Can you work these out from the model? Positions are in its coordinate system, mm. A direction names the side the tool comes from. Coordinates: 2 decimals unless noted, no trailing zeros. Order: outer loops, then holes, each group sorted by start corner. A loop starts at its lowest first (then second) coordinate and runs counter-clockwise, first axis right, second up. Notation, with made-up numbers: (-21.5, -39) -> (4.5, -39) arc R23 cw to (4.5, 0) -> close; hole circle Ø1 at (76.25, -31). An arc over 180 degrees is marked (long way). Answer as CSV lines item,"result".
from build123d import *

# Parameters (mm, degrees)
M10_TAPPED_HOLE1_D           = 8.5
M10_TAPPED_HOLE1_DEPTH       = 24.5
M10_TAPPED_HOLE1_CSINK_D     = 10.05
M10_TAPPED_HOLE1_CSINK_ANGLE = 90
M10_TAPPED_HOLE1_TIP         = 2.553657631
M10_TAPPED_HOLE2_D           = 8.5
M10_TAPPED_HOLE2_DEPTH       = 24.5
M10_TAPPED_HOLE2_CSINK_D     = 10.05
M10_TAPPED_HOLE2_CSINK_ANGLE = 90
M10_TAPPED_HOLE2_TIP         = 2.553657631
CHAMFER1_SIZE                = 1


with BuildPart() as part:
    # Sketch1 → Revolve1 (revolve)
    with BuildSketch(Plane.XY, mode=Mode.PRIVATE) as revolve1_sk:
        Polygon((0, 0), (0, 30), (53.5, 30), (53.5, 32.5), (71.5, 32.5), (71.5, 30), (188, 30), (188, 0), align=None)
    revolve(revolve1_sk.sketch.rotate(Axis((0, 0, 0), (1, 0, 0)), 90), axis=Axis((0, 0, 0), (1, 0, 0)))

    # M10 Tapped Hole1
    with Locations(Plane(origin=(0, 20, 0), x_dir=(0, 0, -1), z_dir=(-1, 0, 0))):
        with Locations((0, 0), (0, 40)):
            CounterSinkHole(M10_TAPPED_HOLE1_D / 2, M10_TAPPED_HOLE1_CSINK_D / 2, depth=M10_TAPPED_HOLE1_DEPTH, counter_sink_angle=M10_TAPPED_HOLE1_CSINK_ANGLE)
            with Locations((0, 0, -(M10_TAPPED_HOLE1_DEPTH + M10_TAPPED_HOLE1_TIP / 2))):  # 118° drill point
                Cone(0, M10_TAPPED_HOLE1_D / 2, M10_TAPPED_HOLE1_TIP, mode=Mode.SUBTRACT)

    # M10 Tapped Hole2
    with Locations(Plane(origin=(188, 20, 0), x_dir=(0, 0, 1), z_dir=(1, 0, 0))):
        with Locations((0, 0), (0, 40)):
            CounterSinkHole(M10_TAPPED_HOLE2_D / 2, M10_TAPPED_HOLE2_CSINK_D / 2, depth=M10_TAPPED_HOLE2_DEPTH, counter_sink_angle=M10_TAPPED_HOLE2_CSINK_ANGLE)
            with Locations((0, 0, -(M10_TAPPED_HOLE2_DEPTH + M10_TAPPED_HOLE2_TIP / 2))):  # 118° drill point
                Cone(0, M10_TAPPED_HOLE2_D / 2, M10_TAPPED_HOLE2_TIP, mode=Mode.SUBTRACT)

    # Chamfer1
    chamfer1_edges = [part.edges().sort_by_distance(p)[0] for p in [
        (0, 0, -30),
        (53.5, 0, -32.5),
        (188, 0, -30),
    ]]
    chamfer(chamfer1_edges, length=CHAMFER1_SIZE)


solid = part.part
Q1. We'd pull the mould along Y, two halves only. Please class faces 4 (the cylindrical face through (27.618, -25.296, 16.128)), 5 (the flat face through (53.5, 12, -28)), 6 (the cylindrical face through (175.2, 24.15, 0.92)): pulls with the +Y half, pulls with the -Y half, needs draft (parallel to the pull), parting line crosses it, or undercut.
Solution:
face 4,"parting line crosses it"
face 5,"needs draft"
face 6,"undercut"
Q2. If I drill on line 1 (Y direction, x = 5.75, z = 0); line 2 (Z direction, x = 172, y = 20); line 3 (Y direction, x = 121, z = -1), over which ranges is the centre line in solid material (lowest first)?
Solution:
line 1,"-30 to -24.25, -15.75 to 15.75, 24.25 to 30"
line 2,"-22.36 to -4.25, 4.25 to 22.36"
line 3,"-29.98 to 29.98"
Q3. Imagine slicing it at A-A (y = 0). List the corners of the cut face in (x, z) for me.
Solution:
outline,"(0, -29) -> (1, -30) -> (53.5, -30) -> (53.5, -31.5) -> (54.5, -32.5) -> (71.5, -32.5) -> (71.5, -30) -> (187, -30) -> (188, -29) -> (188, 29) -> (187, 30) -> (71.5, 30) -> (71.5, 32.5) -> (54.5, 32.5) -> (53.5, 31.5) -> (53.5, 30) -> (1, 30) -> (0, 29) -> close"
Q4. Imagine slicing it at B-B (x = 169). List the corners of the cut face in (y, z) for me, and give its area (3 significant figures).
Solution:
outline,"circle Ø60 at (0, 0); hole circle Ø8.5 at (-20, 0); hole circle Ø8.5 at (20, 0)"
area,"2,710 mm2"
Q5. For P1, Ø1, axis at x = 144.5, y = -9.5, coming from the +Z side; P2, Ø5, axis at y = -20, z = 0, coming from the -X side; P3, Ø6, axis at x = 149, z = -3.5, coming from the -Y side, each with a flat end and sliding along its axis, tell me the tip position at first contact or that it passes through.
Solution:
P1,"z = 28.62"
P2,"x = 25.55"
P3,"y = -30"
Q6. Which directions (+Z, -Z, +X, -X, +Y, -Y) give clear straight access to the entire face, cutting with the end or side of a thin tool? Please do faces 1 (the flat face through (71.5, 29, 9)), 2 (the cylindrical face through (12.8, -15.85, -0.92)), 3 (the flat face through (0, 0, 0)).
Solution:
face 1,"+X"
face 2,"-X"
face 3,"+Z, -Z, -X, +Y, -Y"
